Build history of the part. All positions in model axes, mm. Coordinates: 2 decimals unless noted, no trailing zeros. Loops run counter-clockwise (first coordinate to the right, second up) from the corner with the lowest first, then second, coordinate; pieces in that order, holes last.
(1) Wall check: L1, parallel to Y at x = -3.5, z = -2; L2, parallel to X at y = -67.5, z = 2.5; L3, parallel to X at y = 10.5, z = 8. Give the ranges that are in metal, low to high.
(2) Slice it at A-A (x = 206.5). Give the cut face in (y, z), and give its area (3 significant figures).
(3) Slice it at B-B (y = -40.5). Give the cut face in (x, z), and give its area (3 significant figures).
(4) Flat gauge pins, fed straight in: P1, Ø5, axis at y = 16, z = -4.5, coming from the +X side; P2, Ø2, axis at x = 10.5, z = -0.5, coming from the -Y side; P3, Ø10, axis at y = -24.5, z = -0.5, coming from the -X side. Where does each tip first touch, or does it go through?
from build123d import *

# Parameters (mm, degrees)
F1_W     = 1200
F1_H     = 210
F2_DEPTH = 10
F3_W     = 50
F3_H     = 6.6666666667
F4_DEPTH = 15
F6_DEPTH = 210.001


# Not quite as in the source:
# - a pattern or mirror of a feature is missing from the dataset's text; its kind, count and spacing are read off the source's solid


with BuildPart() as f2:
    # F1 (on Top) → F2 (new body, symmetric)
    with BuildSketch(Plane.XY):
        Rectangle(F1_W, F1_H)
    extrude(amount=F2_DEPTH, both=True)

    # F3 (on face) → F4 (cut)
    with BuildSketch(Plane.XZ.offset(105)):
        Rectangle(F3_W, F3_H)
        with Locations((200, 0)):
            Rectangle(F3_W, F3_H)
        with Locations((400, 0)):
            Rectangle(F3_W, F3_H)
        with Locations((-200, 0)):
            Rectangle(F3_W, F3_H)
        with Locations((-400, 0)):
            Rectangle(F3_W, F3_H)
    f4 = extrude(amount=-F4_DEPTH, mode=Mode.SUBTRACT)

    # F4_copies: F4 across plane
    add(f4.mirror(Plane.ZX), mode=Mode.SUBTRACT)

    # F5 (on face) → F6 (cut, through all)
    with BuildSketch(Plane.XZ.offset(105)):
        Polygon((-421.7155, -10), (-441.7155, 10), (-600, 10), (-600, -10), align=None)
        Polygon((600, -10), (600, 10), (441.7155, 10), (421.7155, -10), align=None)
    extrude(amount=-F6_DEPTH, mode=Mode.SUBTRACT)


solid = f2.part
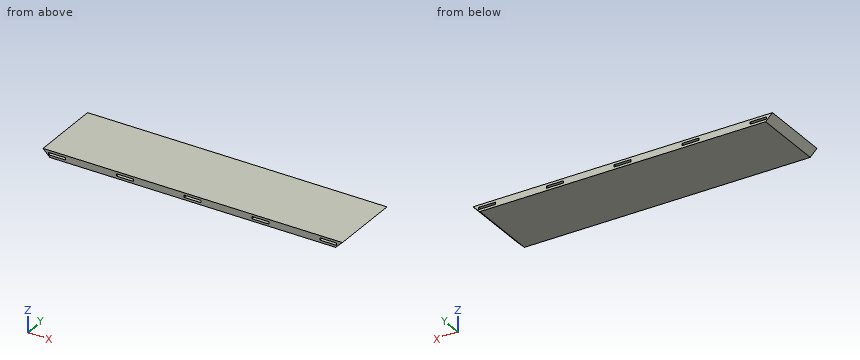
Response values:
1. L1: y = -90 to 90
1. L2: x = -434.22 to 434.22
1. L3: x = -439.72 to 439.72
2. outline: (-105, -10) - (105, -10) - (105, -3.33) - (90, -3.33) - (90, 3.33) - (105, 3.33) - (105, 10) - (-105, 10) - (-105, 3.33) - (-90, 3.33) - (-90, -3.33) - (-105, -3.33) - close
2. area: 4,000 mm2
3. outline: (-441.72, 10) - (-421.72, -10) - (421.72, -10) - (441.72, 10) - close
3. area: 17,300 mm2
4. P1: stops at x = 429.72
4. P2: stops at y = -90
4. P3: stops at x = -436.22
